Answer from the drawing. Dimensions are ordinates in mm from the lowest x, y and z of the part. A direction names the side the tool comes from. Coordinates: 2 decimals unless noted, no trailing zeros. Loops run counter-clockwise (first coordinate to the right, second up) from the corner with the lowest first, then second, coordinate; pieces in that order, holes last. Notation, with made-up numbers: (58.5, -7.5) - (107.5, -7.5) arc R15 cw to (107.5, 21.5) - close; hole circle Ø5 at (-26, 16). An arc over 180 degrees is marked (long way). One line per question, with ' | ' between items. Start each with the question number.
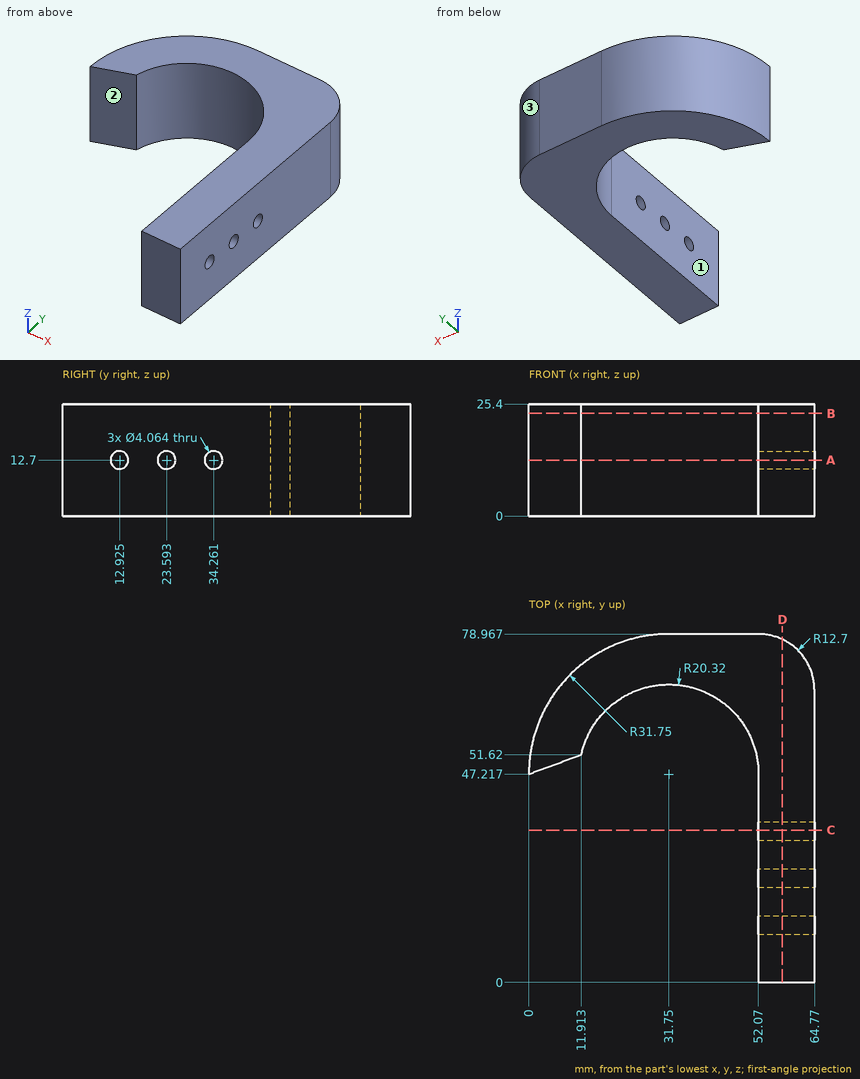
1) The part is cut by section C-C on y = 34.5. Write down the section's boundary in (x, z).
2) The part is cut by section D-D on x = 57.5. Write down the section's boundary in (y, z) (1 decimal), and give its area (3 significant figures).
3) Find the intervals of material crossed by line 1 along X through (y, z) = (43, 21.75); line 2 along X through (y, z) = (57.5, 6) (1 decimal); line 3 along X through (y, z) = (52, 11.75), in increasing order. Write a range as from..to.
4) The part is cut by section A-A on z = 12.7. Count the separate pieces of the cut face and the enclosed holes in it, and give its area (3 significant figures).
5) Which of the six approach directions +Z, -Z, +X, -X, +Y, -Y give full straight-line access (tool end or side, diameter ignored) to the marked faces 1, 2 and 3?
6) The part is cut by section B-B on z = 23.25. Write down the section's boundary in (x, y), and give its area (3 significant figures).
7) Given pin 1 Ø4 at (x, z) = (37, 9.5) entering from -Y; pin 2 Ø5 at (x, z) = (43, 20) entering from -Y; pin 3 Ø6 at (x, z) = (31, 19.5) entering from -Y, each flat-ended and moving along its own axis, determine where each tip first touches the part or whether it passes through.
Answer below:
1) outline: (52.07, 0) - (64.77, 0) - (64.77, 10.68) - (52.07, 10.68) - close; (52.07, 14.72) - (64.77, 14.72) - (64.77, 25.4) - (52.07, 25.4) - close
2) outline: (0, 0) - (77.7, 0) - (77.7, 25.4) - (0, 25.4) - close; hole circle Ø4.1 at (12.9, 12.7); hole circle Ø4.1 at (23.6, 12.7); hole circle Ø4.1 at (34.3, 12.7) | area: 1,940 mm2
3) line 1: 52.07..64.77 | line 2: 1.7..14.2, 49.3..64.8 | line 3: 0.36..12, 51.5..64.77
4) separate pieces: 4 | enclosed holes: 0 | area: 1,580 mm2
5) face 1: +Z, -Z, -X, -Y | face 2: +Z, -Z, -Y | face 3: +Z, -Z, +X, +Y
6) outline: (0, 47.22) - (11.91, 51.62) arc R20.32 cw to (52.07, 47.22) - (52.07, 0) - (64.77, 0) - (64.77, 66.27) arc R12.7 ccw to (52.07, 78.97) - (31.75, 78.97) arc R31.75 ccw to start | area: 1,730 mm2
7) pin 1: y = 66.2 | pin 2: y = 62.18 | pin 3: y = 67.19
